The listing builds one solid part. Answer for the finished solid, in the listing's coordinates (mm). A direction names the side the tool comes from. Coordinates: 2 decimals unless noted, no trailing zeros. Order: outer loops, then holes, each group sorted by start corner. A loop starts at its lowest first (then second) coordinate and runs counter-clockwise, first axis right, second up. Notation, with made-up numbers: (42.5, 66.25) -> (96.5, 66.25) arc R20 ccw to (96.5, 94.25) -> close; hole circle Ø7 at (-11.5, 28). An arc over 180 degrees is marked (long way). Return JSON: item names as keys, results as strings.
```python
from build123d import *

# Parameters (mm, degrees)
F0_R     = 32.004
F1_DEPTH = 4.445
F2_R     = 21.971
F3_DEPTH = 15.748
F4_R     = 1.27
F6_DEPTH = 1.27
F8_DEPTH = 0.508


with BuildPart() as f1:
    # F0 (on Top) → F1 (new body)
    with BuildSketch(Plane.XY):
        with Locations((0.073482, -0.391256)):
            Circle(F0_R)
    extrude(amount=F1_DEPTH)

    # F2 (on face) → F3 (join)
    with BuildSketch(Plane.XY.offset(4.445)):
        Circle(F2_R)
    extrude(amount=F3_DEPTH)

    # F4
    f4_edges = [f1.edges().sort_by_distance(p)[0] for p in [
        (-31.930518, -0.391256, 4.445),
    ]]
    fillet(f4_edges, radius=F4_R)

    # F5 (on face) → F6 (cut)
    with BuildSketch(Plane.XY.offset(20.193)):
        with BuildLine():
            ThreePointArc((-2.289526, -0.856082), (-2.13389, 1.192192), (-0.471214, 2.398492))
            Line((-0.471214, 2.398492), (-0.471214, 3.399117))
            ThreePointArc((-0.471214, 3.399117), (-8.584584, 11.326412), (-1.725764, 20.361088))
            Line((-1.725764, 20.361088), (-2.096043, 20.395772))
            ThreePointArc((-2.096043, 20.395772), (-9.790587, 15.754955), (-12.280816, 7.121187))
            ThreePointArc((-12.280816, 7.121187), (-18.486635, 0.592049), (-18.592949, -8.415199))
            ThreePointArc((-18.592949, -8.415199), (-13.945533, 1.863373), (-3.122954, -1.317712))
            Line((-3.122954, -1.317712), (-2.289526, -0.856082))
        make_face()
        with BuildLine():
            ThreePointArc((7.011916, 8.595588), (-0.036517, 11.09278), (-7.068357, 8.549237))
            Line((-7.068357, 8.549237), (-5.337452, 6.221216))
            ThreePointArc((-5.337452, 6.221216), (-0.035687, 8.19699), (5.28308, 6.267454))
            Line((5.28308, 6.267454), (7.011916, 8.595588))
        make_face()
        with BuildLine():
            ThreePointArc((1.650786, 20.361088), (8.509606, 11.326412), (0.396236, 3.399117))
            Line((0.396236, 3.399117), (0.396236, 2.412013))
            ThreePointArc((0.396236, 2.412013), (2.107861, 1.237631), (2.299367, -0.829289))
            Line((2.299367, -0.829289), (3.040317, -1.287494))
            ThreePointArc((3.040317, -1.287494), (14.022686, 1.79542), (18.381804, -8.745684))
            ThreePointArc((18.381804, -8.745684), (18.472465, 0.397456), (12.227162, 7.075887))
            ThreePointArc((12.227162, 7.075887), (9.947927, 15.477573), (2.680689, 20.270328))
            Line((2.680689, 20.270328), (1.650786, 20.361088))
        make_face()
        with BuildLine():
            Line((10.93796, 1.8472), (8.060673, 1.489116))
            ThreePointArc((8.060673, 1.489116), (7.093825, -4.107257), (2.721723, -7.73202))
            Line((2.721723, -7.73202), (3.911208, -10.380441))
            ThreePointArc((3.911208, -10.380441), (9.617861, -5.527012), (10.93796, 1.8472))
        make_face()
        with BuildLine():
            ThreePointArc((16.792496, -11.514988), (5.471344, -13.055159), (2.636123, -1.987091))
            Line((2.636123, -1.987091), (1.883489, -1.557972))
            ThreePointArc((1.883489, -1.557972), (-0.004876, -2.444337), (-1.889689, -1.550446))
            Line((-1.889689, -1.550446), (-2.723258, -2.012154))
            ThreePointArc((-2.723258, -2.012154), (-5.402938, -12.96385), (-16.620994, -11.834447))
            ThreePointArc((-16.620994, -11.834447), (-8.773086, -16.253179), (-0.014838, -14.153672))
            ThreePointArc((-0.014838, -14.153672), (8.918758, -16.209761), (16.792496, -11.514988))
        make_face()
        with BuildLine():
            Line((-8.065113, 1.464878), (-10.936939, 1.853233))
            ThreePointArc((-10.936939, 1.853233), (-9.638834, -5.490353), (-3.984428, -10.352557))
            Line((-3.984428, -10.352557), (-2.759033, -7.718786))
            ThreePointArc((-2.759033, -7.718786), (-7.097567, -4.100788), (-8.065113, 1.464878))
        make_face()
    extrude(amount=-F6_DEPTH, mode=Mode.SUBTRACT)

    # F7 (on face) → F8 (cut)
    with BuildSketch(Plane(origin=(0, 0, 0), x_dir=(1, 0, 0), z_dir=(0, 0, -1))):
        with BuildLine():
            ThreePointArc((-3.394815, -1.269363), (-3.164044, 1.767733), (-0.698697, 3.556385))
            Line((-0.698697, 3.556385), (-0.698697, 5.04007))
            ThreePointArc((-0.698697, 5.04007), (-12.728867, 16.794335), (-2.558892, 30.190579))
            Line((-2.558892, 30.190579), (-3.107926, 30.242007))
            ThreePointArc((-3.107926, 30.242007), (-14.517077, 23.360795), (-18.209486, 10.559001))
            ThreePointArc((-18.209486, 10.559001), (-27.411217, 0.877866), (-27.568855, -12.477709))
            ThreePointArc((-27.568855, -12.477709), (-20.677859, 2.762933), (-4.630586, -1.953849))
            Line((-4.630586, -1.953849), (-3.394815, -1.269363))
        make_face()
        with BuildLine():
            ThreePointArc((10.396979, 12.745183), (-0.054146, 16.447916), (-10.480667, 12.676454))
            Line((-10.480667, 12.676454), (-7.914152, 9.224561))
            ThreePointArc((-7.914152, 9.224561), (-0.052915, 12.154157), (7.833533, 9.293121))
            Line((7.833533, 9.293121), (10.396979, 12.745183))
        make_face()
        with BuildLine():
            ThreePointArc((2.447718, 30.190579), (12.617692, 16.794335), (0.587522, 5.04007))
            Line((0.587522, 5.04007), (0.587522, 3.576432))
            ThreePointArc((0.587522, 3.576432), (3.125449, 1.835108), (3.409406, -1.229636))
            Line((3.409406, -1.229636), (4.508056, -1.909044))
            ThreePointArc((4.508056, -1.909044), (20.792258, 2.662175), (27.255778, -12.967738))
            ThreePointArc((27.255778, -12.967738), (27.390206, 0.589332), (18.129931, 10.491833))
            ThreePointArc((18.129931, 10.491833), (14.750374, 22.949505), (3.974815, 30.056004))
            Line((3.974815, 30.056004), (2.447718, 30.190579))
        make_face()
        with BuildLine():
            Line((16.218354, 2.738951), (11.952032, 2.208))
            ThreePointArc((11.952032, 2.208), (10.51843, -6.090071), (4.035658, -11.46472))
            Line((4.035658, -11.46472), (5.799377, -15.391689))
            ThreePointArc((5.799377, -15.391689), (14.260966, -8.195225), (16.218354, 2.738951))
        make_face()
        with BuildLine():
            ThreePointArc((24.899218, -17.073947), (8.112683, -19.35765), (3.908734, -2.946376))
            Line((3.908734, -2.946376), (2.79276, -2.310096))
            ThreePointArc((2.79276, -2.310096), (-0.007229, -3.624362), (-2.801953, -2.298937))
            Line((-2.801953, -2.298937), (-4.037934, -2.983539))
            ThreePointArc((-4.037934, -2.983539), (-8.011253, -19.222261), (-24.644922, -17.547628))
            ThreePointArc((-24.644922, -17.547628), (-13.008369, -24.099542), (-0.022, -20.986479))
            ThreePointArc((-0.022, -20.986479), (13.224366, -24.035163), (24.899218, -17.073947))
        make_face()
        with BuildLine():
            Line((-11.958616, 2.17206), (-16.216841, 2.747898))
            ThreePointArc((-16.216841, 2.747898), (-14.292065, -8.140869), (-5.907945, -15.350344))
            Line((-5.907945, -15.350344), (-4.09098, -11.445096))
            ThreePointArc((-4.09098, -11.445096), (-10.523978, -6.080479), (-11.958616, 2.17206))
        make_face()
    extrude(amount=-F8_DEPTH, mode=Mode.SUBTRACT)


solid = f1.part
```
Item 1: Find the intervals of material crossed by probe 1 along X at (y, z) = (18, 19.75); probe 2 along Z at (x, y) = (22, -13) (3 decimals); probe 3 along Z at (x, y) = (-1, -8.5), in increasing order.
Answer list:
{"probe 1": "-12.6 to -7.55, -6.12 to 6.04, 7.5 to 12.6", "probe 2": "0 to 4.445", "probe 3": "0 to 18.92"}
Item 2: Determine the mould class of faces 1 (the cylindrical face through (-5.26, -12.86, 19.57)), 2 (the cylindrical face through (-6.864, -31.634, 1.565)), 3 (the flat face through (0, 0, 20.193)) for opening direction Y: pulls with the +Y half, pulls with the -Y half, needs draft (parallel to the pull), parting line crosses it, or undercut.
Answer list:
{"face 1": "undercut", "face 2": "parting line crosses it", "face 3": "needs draft"}
Item 3: The part is cut by section A-A on z = 16.5. Determine the outline of the cut face in (x, y), plus the area to 3 significant figures.
Answer list:
{"outline": "circle Ø43.94 at (0, 0)", "area": "1,520 mm2"}
Item 4: Which of the six approach directions +Z, -Z, +X, -X, +Y, -Y give full straight-line access (tool end or side, diameter ignored) to faces 4 (the flat face through (-15, -7, 0.508)), 5 (the cylindrical face through (10.02, 15.38, 19.57)), 6 (the flat face through (0, 0, 0))?
Answer list:
{"face 4": "-Z", "face 5": "+Z", "face 6": "-Z, +X, -X, +Y, -Y"}
Item 5: Flat-ended cylindrical pins translate along their axes: pin 1 (6 mm diameter, centred on y = 9, z = 7.5, fed in from -X); pin 2 (12 mm diameter, centred on y = 15, z = 14, fed in from +X); pin 3 (2.5 mm diameter, centred on x = 1, y = 9.5, fed in from +Z). Find the tip coordinate at first contact, or state that the pin passes through.
Answer list:
{"pin 1": "x = -21.14", "pin 2": "x = 20.04", "pin 3": "z = 18.92"}
